The drawing under review shows one solid part. Ordinate dimensions are in mm from its lowest x, y, z. A direction names the side the tool comes from. Give positions to 0.01 mm unless a question says otherwise; leave off trailing zeros. Loops run counter-clockwise (first coordinate to the right, second up) from the corner with the lowest first, then second, coordinate; pieces in that order, holes last. Notation, with made-up numbers: M 49,57 L 65,57 A17 cw 65,88 Z; hole C -11,18 d8. An arc over 180 degrees is marked long. Answer as CSV lines item,"result".
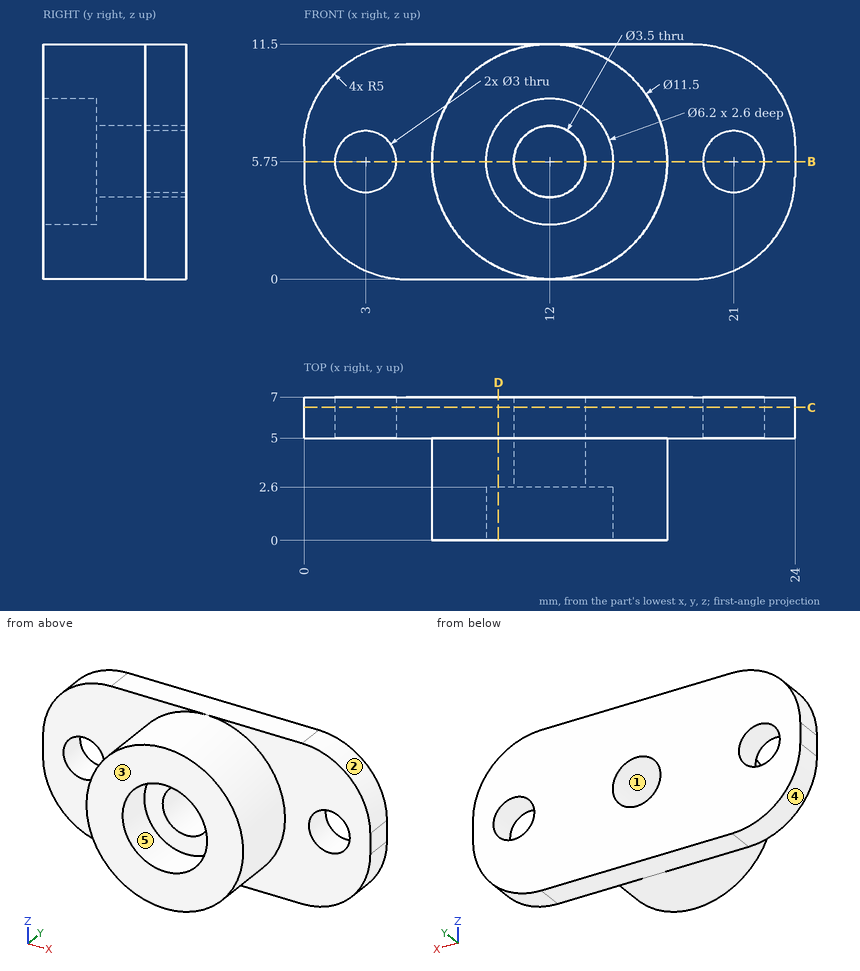
1. We need section B-B, the plane z = 5.75. Write out the cut boundary in (x, y).
Answer block:
outline,"M 0,5 L 1.5,5 L 1.5,7 L 0,7 Z; M 4.5,5 L 6.25,5 L 6.25,0 L 8.9,0 L 8.9,2.6 L 10.25,2.6 L 10.25,7 L 4.5,7 Z; M 13.75,2.6 L 15.1,2.6 L 15.1,0 L 17.75,0 L 17.75,5 L 19.5,5 L 19.5,7 L 13.75,7 Z; M 22.5,5 L 24,5 L 24,7 L 22.5,7 Z"
2. For the marked faces 4 and 5, list the 3-axis set-ups (+Z, -Z, +X, -X, +Y, -Y) from which the entire face can be reached by the end or side of a thin tool; tool diameter is ignored.
Answer block:
face 4,"-Z, -X, +Y, -Y"
face 5,"-Y"
3. The part is to be moulded in two halves that separate along Z. For the marked faces 1, 2 and 3, say which applies: pulls with the +Z half, pulls with the -Z half, needs draft (parallel to the pull), parting line crosses it, or undercut.
Answer block:
face 1,"undercut"
face 2,"pulls with the +Z half"
face 3,"needs draft"
4. We need section D-D, the plane x = 9.5. Write out the cut boundary in (y, z).
Answer block:
outline,"M 0,0.57 L 5,0.57 L 5,0 L 7,0 L 7,11.5 L 5,11.5 L 5,10.93 L 0,10.93 L 0,7.58 L 2.6,7.58 L 2.6,3.92 L 0,3.92 Z"
5. We need section C-C, the plane y = 6.5. Write out the cut boundary in (x, z), plus the area to 3 significant figures.
Answer block:
outline,"M 0,5 A5 ccw 5,0 L 19,0 A5 ccw 24,5 L 24,6.5 A5 ccw 19,11.5 L 5,11.5 A5 ccw 0,6.5 Z; hole C 3,5.75 d3; hole C 12,5.75 d3.5; hole C 21,5.75 d3"
area,"231 mm²"
6. For P1, Ø4, axis at x = 21, z = 5.75, coming from the -Y side; P2, Ø5.5, axis at x = 12, z = 5.75, coming from the +Y side, all flat-tipped, find the tip position at first contact; note any pin that passes through.
Answer block:
P1,"y = 5"
P2,"y = 7"
7. To check wall thickness, follow L1, parallel to X at y = 6.25, z = 5.75; L2, parallel to X at y = 4.35, z = 5.75; L3, parallel to Z at x = 12, y = 5.85. State the ranges of each line that lie inside material, in increasing order. Write a range as [from, to].
Answer block:
L1,"[0, 1.5], [4.5, 10.25], [13.75, 19.5], [22.5, 24]"
L2,"[6.25, 10.25], [13.75, 17.75]"
L3,"[0, 4], [7.5, 11.5]"
